Can you work these out from the model? Positions are in its coordinate system, mm. Face numbers are marked on the shaded views. A direction names the side the tool comes from. Round coordinates to 2 decimals unless told otherwise and drop trailing zeros. Write each loop counter-clockwise with the first axis right and the second up, starting at its lowest first coordinate (ties: lowest second). Pieces come first, ordered by that corner, then holes. Notation, with made-up numbers: (-10, 22) -> (19, 22) arc R15 cw to (19, 37) -> close; hole circle Ø1 at (9, -24). An arc over 180 degrees is marked (long way). Write item = value, one per line. Start each with the question number.
1) Imagine slicing it at C-C, the plane x = 0. Please give me the cut outline in (y, z), then the cut area to 3 significant figures.
2) If I drill on line 1 (X direction, y = -1.6, z = 5.75); line 2 (X direction, y = 0.1, z = 11.5); line 3 (Y direction, x = 0, z = 3), over which ranges is the centre line in solid material (lowest first)?
3) Thinking about a two-plate mould opening in X: for the marked faces 4, 5, 6 and 7, which applies, +X half, -X half, draft (parallel to the pull), parting line (faces both ways), or undercut?
4) Imagine slicing it at A-A, the plane y = -1.05. Please give me the cut outline in (x, z).
5) For the marked faces 1, 2 and 3, which set-ups out of +Z, -Z, +X, -X, +Y, -Y let a thin tool reach every point of the face, with its end or its side?
6) I'm going to push flat-ended pins straight in: pin 1 (1.3 mm diameter, centred on x = 5, z = 8, fed in from +Y); pin 2 (3 mm diameter, centred on x = -5, z = 3, fed in from +Y); pin 3 (6 mm diameter, centred on x = 4.5, z = 6, fed in from +Y). Where does each tip first touch, or does it pass through?
7) Imagine slicing it at D-D, the plane y = 1.6. Please give me the cut outline in (x, z).
8) Imagine slicing it at B-B, the plane z = 7.25. Please give me the cut outline in (x, y).
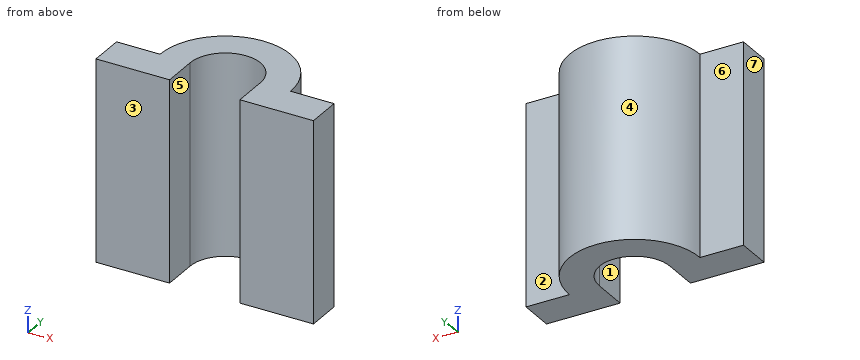
from build123d import *

# Parameters (mm, degrees)
BOSS_EXTRUDE1_DEPTH = 12


with BuildPart() as part:
    # Sketch1 → Boss-Extrude1 (new body)
    with BuildSketch(Plane.XY):
        with BuildLine():
            Line((-2.1, 0), (-2.1, -2.1))
            Line((-2.1, -2.1), (-6.5, -2.1))
            Line((-6.5, -2.1), (-6.5, 0))
            Line((-6.5, 0), (-3.9, 0))
            ThreePointArc((-3.9, 0), (0, 3.9), (3.9, 0))
            Line((3.9, 0), (6.5, 0))
            Line((6.5, 0), (6.5, -2.1))
            Line((6.5, -2.1), (2.1, -2.1))
            Line((2.1, -2.1), (2.1, 0))
            ThreePointArc((2.1, 0), (0, 2.1), (-2.1, 0))
        make_face()
    extrude(amount=BOSS_EXTRUDE1_DEPTH)


solid = part.part
Reported:
q1.outline = (2.1, 0) -> (3.9, 0) -> (3.9, 12) -> (2.1, 12) -> close
q1.area = 21.6 mm²
q2.line_1 = -6.5 to -2.1, 2.1 to 6.5
q2.line_2 = -3.9 to -2.1, 2.1 to 3.9
q2.line_3 = 2.1 to 3.9
q3.face_4 = parting line
q3.face_5 = undercut
q3.face_6 = draft
q3.face_7 = -X half
q4.outline = (-6.5, 0) -> (-2.1, 0) -> (-2.1, 12) -> (-6.5, 12) -> close; (2.1, 0) -> (6.5, 0) -> (6.5, 12) -> (2.1, 12) -> close
q5.face_1 = +Z, -Z, -Y
q5.face_2 = +Z, -Z, +X, +Y
q5.face_3 = +Z, -Z, +X, -X, -Y
q6.pin_1 = 0
q6.pin_2 = 1.72
q6.pin_3 = 3.6
q7.outline = (-3.56, 0) -> (-1.36, 0) -> (-1.36, 12) -> (-3.56, 12) -> close; (1.36, 0) -> (3.56, 0) -> (3.56, 12) -> (1.36, 12) -> close
q8.outline = (-6.5, -2.1) -> (-2.1, -2.1) -> (-2.1, 0) arc R2.1 cw to (2.1, 0) -> (2.1, -2.1) -> (6.5, -2.1) -> (6.5, 0) -> (3.9, 0) arc R3.9 ccw to (-3.9, 0) -> (-6.5, 0) -> close
